Can you work these out from the model? Positions are in its coordinate system, mm. Coordinates: 2 decimals unless noted, no trailing zeros. Order: outer loops, then holes, each group sorted by start corner. A loop starts at its lowest first (then second) coordinate and runs counter-clockwise, first axis right, second up. Notation, with made-up numbers: (-7.5, 57.25) - (15.5, 57.25) arc R21 cw to (15.5, 68.25) - close; hole circle Ø3 at (23, 9.25). An arc over 180 degrees is marked (long way). Return JSON: item names as keys, results as strings. Group by question number.
1) If I drill on line 1 along X through (y, z) = (0.5, 1); line 2 along X through (y, z) = (0.65, -18.5); line 3 along X through (y, z) = (0.75, -1.5), over which ranges is the centre line in solid material (lowest first)?
2) Imagine slicing it at B-B (x = 37.5). Write out the boundary of the cut face in (y, z).
3) Imagine slicing it at A-A (x = -44). Write out the boundary of the cut face in (y, z).
4) Imagine slicing it at C-C (y = 1.15). Give the number of separate pieces and of enclosed holes in the cut face, and give its area (3 significant figures).
5) For pin 1 Ø2.5 at (x, z) = (-59.7, -28.2) entering from +Y; pin 2 Ø1.2 at (x, z) = (19.5, -27.8) entering from -Y; pin 3 Ø0.8 at (y, z) = (1, -1) entering from +X (3 decimals), each with a flat end and sliding along its axis, tell me the tip position at first contact or that it passes through.
```python
from build123d import *

# Parameters (mm, degrees)
ESBO_O1_W                          = 131.4
ESBO_O1_H                          = 68.4
BASE_DEPTH                         = 1.5
FILETE1_R                          = 10
FILETE2_R                          = 10
FILETE3_R                          = 15
FILETE4_R                          = 15
ESBO_O2_R                          = 6.2
FURO_DOS_BOT_ES_DEPTH              = 75.083601424
DISPLAY_START                      = -1.5
DISPLAY_OUTLINE_W                  = 24
DISPLAY_OUTLINE_H                  = 3
DISPLAY_DEPTH                      = 1.5
FILETE5_R                          = 1
FURO_BUZZER_DEPTH                  = 75.083601424
ESBO_O5_R                          = 1
FURO_DOS_PARAFUSOS_DEPTH           = 75.083601424
ESBO_O6_R                          = 2.5
FURO_DA_CABE_A_DOS_PARAFUSOS_DEPTH = 0.6
ESBO_O7_R                          = 1
FURO_ADICIONAIS_DO_DISPLAY_DEPTH   = 10


# Read off the part's stored shape, not the designer's step: Display
with BuildPart() as part:
    # Esboço1 → Base (new body)
    with BuildSketch(Plane(origin=(0, 0, 0), x_dir=(1, 0, 0), z_dir=(0, 1, 0))):
        Rectangle(ESBO_O1_W, ESBO_O1_H)
    extrude(amount=BASE_DEPTH)

    # Filete1
    filete1_edges = [part.edges().sort_by_distance(p)[0] for p in [
        (65.7, 0.75, -34.2),
    ]]
    fillet(filete1_edges, radius=FILETE1_R)

    # Filete2
    filete2_edges = [part.edges().sort_by_distance(p)[0] for p in [
        (-65.7, 0.75, -34.2),
    ]]
    fillet(filete2_edges, radius=FILETE2_R)

    # Filete3
    filete3_edges = [part.edges().sort_by_distance(p)[0] for p in [
        (-65.7, 0.75, 34.2),
    ]]
    fillet(filete3_edges, radius=FILETE3_R)

    # Filete4
    filete4_edges = [part.edges().sort_by_distance(p)[0] for p in [
        (65.7, 0.75, 34.2),
    ]]
    fillet(filete4_edges, radius=FILETE4_R)

    # Esboço2 → Furo dos botões (cut, through all)
    with BuildSketch(Plane(origin=(0, 1.5, 0), x_dir=(1, 0, 0), z_dir=(0, 1, 0))):
        with Locations(Location((-44, -1, 0), (0, 0, 270))):
            Circle(ESBO_O2_R)
        with Locations(Location((-32.5, -12.5, 0), (0, 0, 270))):
            Circle(ESBO_O2_R)
        with Locations(Location((-55.5, -12.5, 0), (0, 0, 270))):
            Circle(ESBO_O2_R)
        with Locations(Location((-44, -24, 0), (0, 0, 270))):
            Circle(ESBO_O2_R)
        with Locations(Location((37.5, -24, 0), (0, 0, 270))):
            Circle(ESBO_O2_R)
        with Locations(Location((49, -12.5, 0), (0, 0, 270))):
            Circle(ESBO_O2_R)
        with Locations(Location((10.3, -24, 0), (0, 0, 270))):
            Circle(ESBO_O2_R)
    extrude(amount=-FURO_DOS_BOT_ES_DEPTH, mode=Mode.SUBTRACT)

    # Display outline → Display (cut)
    with BuildSketch(Plane(origin=(0, 1.5, 0), x_dir=(1, 0, 0), z_dir=(0, 1, 0)).offset(DISPLAY_START)):
        with Locations((-1, -13)):
            Rectangle(DISPLAY_OUTLINE_W, DISPLAY_OUTLINE_H)
    extrude(amount=DISPLAY_DEPTH, mode=Mode.SUBTRACT)

    # Filete5
    filete5_edges = [part.edges().sort_by_distance(p)[0] for p in [
        (0, 1.5, -34.2),
        (62.771067812, 1.5, -31.271067812),
        (-65.7, 1.5, -2.5),
        (-62.771067812, 1.5, -31.271067812),
        (0, 1.5, 34.2),
        (-61.306601718, 1.5, 29.806601718),
        (65.7, 1.5, -2.5),
        (61.306601718, 1.5, 29.806601718),
    ]]
    fillet(filete5_edges, radius=FILETE5_R)

    # Esboço4 → Furo buzzer (cut, through all)
    with BuildSketch(Plane(origin=(0, 1.5, 0), x_dir=(1, 0, 0), z_dir=(0, 1, 0))):
        with BuildLine():
            Line((-11.223401872, -20.676598128), (-9.809188309, -22.090811691))
            Line((-9.809188309, -22.090811691), (-8.041421356, -20.323044738))
            ThreePointArc((-8.041421356, -20.323044738), (-8.041421356, -18.908831175), (-9.455634919, -18.908831175))
            Line((-9.455634919, -18.908831175), (-11.223401872, -20.676598128))
        make_face()
        with BuildLine():
            Line((-11.576955262, -23.858578644), (-9.809188309, -22.090811691))
            Line((-9.809188309, -22.090811691), (-11.223401872, -20.676598128))
            Line((-11.223401872, -20.676598128), (-12.991168825, -22.444365081))
            ThreePointArc((-12.991168825, -22.444365081), (-12.991168825, -23.858578644), (-11.576955262, -23.858578644))
        make_face()
        with BuildLine():
            Line((-5.460481605, -19.86342533), (-8.748528137, -23.151471863))
            Line((-8.748528137, -23.151471863), (-7.051471863, -24.848528137))
            Line((-7.051471863, -24.848528137), (-3.76342533, -21.560481605))
            ThreePointArc((-3.76342533, -21.560481605), (-3.76342533, -19.86342533), (-5.460481605, -19.86342533))
        make_face()
        with BuildLine():
            Line((-8.748528137, -23.151471863), (-12.03657467, -26.439518395))
            ThreePointArc((-12.03657467, -26.439518395), (-12.03657467, -28.13657467), (-10.339518395, -28.13657467))
            Line((-10.339518395, -28.13657467), (-7.051471863, -24.848528137))
            Line((-7.051471863, -24.848528137), (-8.748528137, -23.151471863))
        make_face()
        with BuildLine():
            Line((-4.576598128, -27.323401872), (-5.990811691, -25.909188309))
            Line((-5.990811691, -25.909188309), (-7.758578644, -27.676955262))
            ThreePointArc((-7.758578644, -27.676955262), (-7.758578644, -29.091168825), (-6.344365081, -29.091168825))
            Line((-6.344365081, -29.091168825), (-4.576598128, -27.323401872))
        make_face()
        with BuildLine():
            Line((-4.223044738, -24.141421356), (-5.990811691, -25.909188309))
            Line((-5.990811691, -25.909188309), (-4.576598128, -27.323401872))
            Line((-4.576598128, -27.323401872), (-2.808831175, -25.555634919))
            ThreePointArc((-2.808831175, -25.555634919), (-2.808831175, -24.141421356), (-4.223044738, -24.141421356))
        make_face()
    extrude(amount=-FURO_BUZZER_DEPTH, mode=Mode.SUBTRACT)

    # Esboço5 → Furo dos parafusos (cut, through all)
    with BuildSketch(Plane(origin=(0, 1.5, 0), x_dir=(1, 0, 0), z_dir=(0, 1, 0))):
        with Locations(Location((59.7, 28.2, 0), (0, 0, 270))):
            Circle(ESBO_O5_R)
        with Locations(Location((57.7, -26.2, 0), (0, 0, 270))):
            Circle(ESBO_O5_R)
        with Locations(Location((-57.7, -26.2, 0), (0, 0, 270))):
            Circle(ESBO_O5_R)
        with Locations(Location((-59.7, 28.2, 0), (0, 0, 270))):
            Circle(ESBO_O5_R)
    extrude(amount=-FURO_DOS_PARAFUSOS_DEPTH, mode=Mode.SUBTRACT)

    # Esboço6 → Furo da cabeça dos parafusos (cut)
    with BuildSketch(Plane(origin=(0, 1.5, 0), x_dir=(1, 0, 0), z_dir=(0, 1, 0))):
        with Locations(Location((-59.7, 28.2, 0), (0, 0, 270))):
            Circle(ESBO_O6_R)
        with Locations(Location((59.7, 28.2, 0), (0, 0, 270))):
            Circle(ESBO_O6_R)
        with Locations(Location((57.7, -26.2, 0), (0, 0, 270))):
            Circle(ESBO_O6_R)
        with Locations(Location((-57.7, -26.2, 0), (0, 0, 270))):
            Circle(ESBO_O6_R)
    extrude(amount=-FURO_DA_CABE_A_DOS_PARAFUSOS_DEPTH, mode=Mode.SUBTRACT)

    # Esboço7 → Furo adicionais do display (cut)
    with BuildSketch(Plane(origin=(0, 1.5, 0), x_dir=(1, 0, 0), z_dir=(0, 1, 0))):
        with Locations(Location((-21.5, -13, 0), (0, 0, 270))):
            Circle(ESBO_O7_R)
        with Locations(Location((19.5, -13, 0), (0, 0, 270))):
            Circle(ESBO_O7_R)
        with Locations(Location((-21.5, 27.8, 0), (0, 0, 270))):
            Circle(ESBO_O7_R)
        with Locations(Location((19.5, 27.8, 0), (0, 0, 270))):
            Circle(ESBO_O7_R)
        with BuildLine():
            Line((-22.75, -1.5), (-22.75, 2.5))
            ThreePointArc((-22.75, 2.5), (-21.5, 3.75), (-20.25, 2.5))
            Line((-20.25, 2.5), (-20.25, -1.5))
            ThreePointArc((-20.25, -1.5), (-21.5, -2.75), (-22.75, -1.5))
        make_face()
        with BuildLine():
            Line((-22.75, 19.3), (-22.75, 23.3))
            ThreePointArc((-22.75, 23.3), (-21.5, 24.55), (-20.25, 23.3))
            Line((-20.25, 23.3), (-20.25, 19.3))
            ThreePointArc((-20.25, 19.3), (-21.5, 18.05), (-22.75, 19.3))
        make_face()
        with BuildLine():
            Line((18.25, 19.3), (18.25, 23.3))
            ThreePointArc((18.25, 23.3), (19.5, 24.55), (20.75, 23.3))
            Line((20.75, 23.3), (20.75, 19.3))
            ThreePointArc((20.75, 19.3), (19.5, 18.05), (18.25, 19.3))
        make_face()
        with BuildLine():
            Line((18.25, -1.5), (18.25, 2.5))
            ThreePointArc((18.25, 2.5), (19.5, 3.75), (20.75, 2.5))
            Line((20.75, 2.5), (20.75, -1.5))
            ThreePointArc((20.75, -1.5), (19.5, -2.75), (18.25, -1.5))
        make_face()
    extrude(amount=-FURO_ADICIONAIS_DO_DISPLAY_DEPTH, mode=Mode.SUBTRACT)


solid = part.part
```
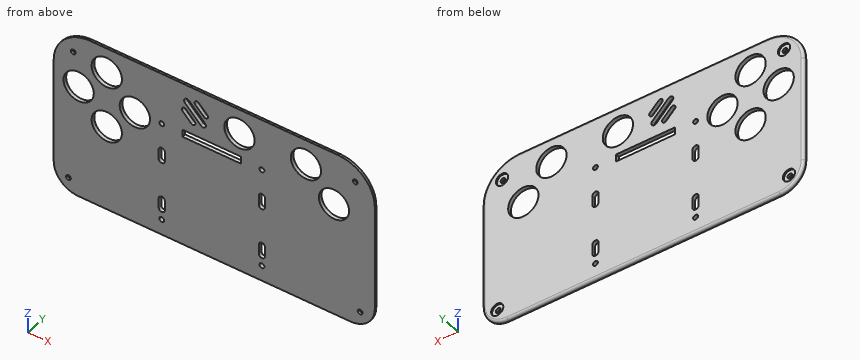
Calculated:
{
 "1": {"line 1": "-65.7 to -50.2, -37.8 to -22.75, -20.25 to 18.25, 20.75 to 65.7", "line 2": "-65.69 to -22.46, -20.54 to 18.54, 20.46 to 65.69", "line 3": "-65.67 to -49.67, -38.33 to -22.75, -20.25 to 18.25, 20.75 to 65.67"},
 "2": {"outline": "(0, -34.2) - (0.5, -34.2) arc R1 ccw to (1.5, -33.2) - (1.5, 17.8) - (0, 17.8) - close; (0, 30.2) - (1.5, 30.2) - (1.5, 33.2) arc R1 ccw to (0.5, 34.2) - (0, 34.2) - close"},
 "3": {"outline": "(0, -34.2) - (0.5, -34.2) arc R1 ccw to (1.5, -33.2) - (1.5, -5.2) - (0, -5.2) - close; (0, 7.2) - (1.5, 7.2) - (1.5, 17.8) - (0, 17.8) - close; (0, 30.2) - (1.5, 30.2) - (1.5, 33.2) arc R1 ccw to (0.5, 34.2) - (0, 34.2) - close"},
 "4": {"separate pieces": "1", "enclosed holes": "23", "area": "7,640 mm2"},
 "5": {"pin 1": "y = 0.9", "pin 2": "through", "pin 3": "x = 65.695"}
}
